Geometry check sheet. Reference: the model listing, model coordinates, mm. Face numbers are marked on the shaded views. A direction names the side the tool comes from. Give positions to 0.01 mm unless a question says otherwise; leave off trailing zeros. Order: outer loops, then holes, each group sorted by start corner. A loop starts at its lowest first (then second) coordinate and runs counter-clockwise, first axis right, second up. Notation, with made-up numbers: M -24.75,58.5 L -7.75,58.5 A17 ccw -7.75,73.5 Z; hole C 55,-0.5 d11. An arc over 180 degrees is marked long. One line per question, with ' | ' between items. Start each with the question number.
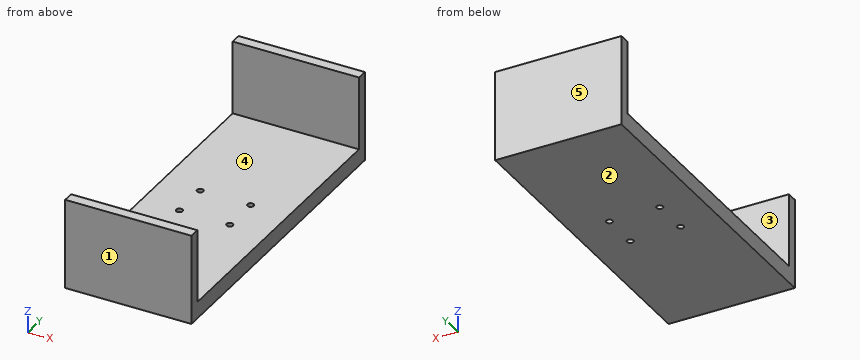
from build123d import *

# Parameters (mm, degrees)
SKETCH2_W           = 60
SKETCH2_H           = 150
SKETCH2_R           = 1.5
BOSS_EXTRUDE1_DEPTH = 8
SKETCH5_W           = 60
SKETCH5_H           = 5.066428815
BOSS_EXTRUDE2_DEPTH = 35


with BuildPart() as part:
    # Sketch2 → Boss-Extrude1 (new body)
    with BuildSketch(Plane.XY):
        with Locations((16.635, 15)):
            Rectangle(SKETCH2_W, SKETCH2_H)
        with Locations((28.6, 24.016821687)):
            Circle(SKETCH2_R, mode=Mode.SUBTRACT)
        with Locations(Location((28.6, 5.983178313, 0), (0, 0, 180))):
            Circle(SKETCH2_R, mode=Mode.SUBTRACT)
        with Locations((4.67, 5.983178313)):
            Circle(SKETCH2_R, mode=Mode.SUBTRACT)
        with Locations(Location((4.67, 24.016821687, 0), (0, 0, 180))):
            Circle(SKETCH2_R, mode=Mode.SUBTRACT)
    extrude(amount=BOSS_EXTRUDE1_DEPTH)

    # Sketch5 → Boss-Extrude2 (add)
    with BuildSketch(Plane.XY.offset(8)):
        with Locations((16.635, 87.466785593)):
            Rectangle(SKETCH5_W, SKETCH5_H)
        with Locations((16.635, -57.466785593)):
            Rectangle(SKETCH5_W, SKETCH5_H)
    extrude(amount=BOSS_EXTRUDE2_DEPTH)


solid = part.part
Item 1: Cross-section at A-A, the plane x = 4.67. Record the cut outline in (y, z).
Item 2: Material ranges on line 1 along Y through (x, z) = (28.6, 4); line 2 along Y through (x, z) = (28, 6); line 3 along Y through (x, z) = (44, 32), recorded low to high.
Item 3: Cross-section at B-B, the plane z = 29.5. Record the cut outline in (x, y) (3 decimals), plus the area to 3 significant figures.
Item 4: Depth check by flat-ended pin: pin 1 (3 mm diameter, centred on x = 30, y = -8.5, fed in from +Z); pin 2 (2.5 mm diameter, centred on x = 28.6, y = 24.02, fed in from +Z). Enter the tip coordinate at first touch or a pass-through.
Item 5: Set-up check for the marked faces 4 and 5: record each of +Z, -Z, +X, -X, +Y, -Y from which the full face is reachable in a straight line by a thin tool's end or side.
Item 6: Cross-section at C-C, the plane x = -2.5. Record the cut outline in (y, z), plus the area to 3 significant figures.
Item 7: Mould release check, pull along Y, two halves, no side actions. Record for the marked faces 1, 2 and 3: released by +Y, released by -Y, zero draft, split by the parting line, or undercut.
Item 8: Cross-section at D-D, the plane y = 76.5. Record the cut outline in (x, z) (3 decimals), plus the area to 3 significant figures.
Outcome:
1) outline: M -60,0 L 4.48,0 L 4.48,8 L -54.93,8 L -54.93,43 L -60,43 Z; M 7.48,0 L 22.52,0 L 22.52,8 L 7.48,8 Z; M 25.52,0 L 90,0 L 90,43 L 84.93,43 L 84.93,8 L 25.52,8 Z
2) line 1: y = -60 to 4.48, 7.48 to 22.52, 25.52 to 90 | line 2: y = -60 to 4.61, 7.36 to 22.64, 25.39 to 90 | line 3: y = -60 to -54.93, 84.93 to 90
3) outline: M -13.365,-60 L 46.635,-60 L 46.635,-54.934 L -13.365,-54.934 Z; M -13.365,84.934 L 46.635,84.934 L 46.635,90 L -13.365,90 Z | area: 608 mm²
4) pin 1: stops at z = 8 | pin 2: passes through
5) face 4: +Z, +X, -X | face 5: +Z, -Z, +X, -X, +Y
6) outline: M -60,0 L 90,0 L 90,43 L 84.93,43 L 84.93,8 L -54.93,8 L -54.93,43 L -60,43 Z | area: 1,550 mm²
7) face 1: released by -Y | face 2: zero draft | face 3: undercut
8) outline: M -13.365,0 L 46.635,0 L 46.635,8 L -13.365,8 Z | area: 480 mm²
